```python
from build123d import *

# Parameters (mm, degrees)
SKETCH1_W           = 361.95
SKETCH1_H           = 460.375
BOSS_EXTRUDE1_DEPTH = 3.175
SKETCH2_W           = 3.175
SKETCH2_H           = 82.55
SKETCH2_H_2         = 44.45
SKETCH2_W_2         = 22.225
SKETCH2_H_3         = 3.175
CUT_EXTRUDE1_DEPTH  = 3.175
SKETCH3_R           = 12.0777
CUT_EXTRUDE2_DEPTH  = 3.175


with BuildPart() as part:
    # Sketch1 → Boss-Extrude1 (new body)
    with BuildSketch(Plane(origin=(0, 0, 0), x_dir=(0, 0, -1), z_dir=(1, 0, 0))):
        with Locations((0, 230.1875)):
            Rectangle(SKETCH1_W, SKETCH1_H)
    extrude(amount=BOSS_EXTRUDE1_DEPTH)

    # Sketch2 → Cut-Extrude1 (cut)
    with BuildSketch(Plane(origin=(3.175, 0, 0), x_dir=(0, 0, -1), z_dir=(1, 0, 0))):
        with Locations((-179.3875, 41.275)):
            Rectangle(SKETCH2_W, SKETCH2_H)
        with Locations((-179.3875, 180.975)):
            Rectangle(SKETCH2_W, SKETCH2_H_2)
        with Locations((-179.3875, 301.625)):
            Rectangle(SKETCH2_W, SKETCH2_H_2)
        Polygon((-98.425, 460.375), (-180.975, 460.375), (-180.975, 400.05), (-177.8, 400.05), (-177.8, 457.2), (-98.425, 457.2), align=None)
        with Locations((-11.1125, 458.7875)):
            Rectangle(SKETCH2_W_2, SKETCH2_H_3)
        with Locations((11.1125, 458.7875)):
            Rectangle(SKETCH2_W_2, SKETCH2_H_3)
        Polygon((180.975, 460.375), (98.425, 460.375), (98.425, 457.2), (177.8, 457.2), (177.8, 400.05), (180.975, 400.05), align=None)
        with Locations((179.3875, 301.625)):
            Rectangle(SKETCH2_W, SKETCH2_H_2)
        with Locations((179.3875, 180.975)):
            Rectangle(SKETCH2_W, SKETCH2_H_2)
        with Locations((179.3875, 41.275)):
            Rectangle(SKETCH2_W, SKETCH2_H)
    extrude(amount=-CUT_EXTRUDE1_DEPTH, mode=Mode.SUBTRACT)

    # Sketch3 → Cut-Extrude2 (cut)
    with BuildSketch(Plane(origin=(3.175, 0, 0), x_dir=(0, 0, -1), z_dir=(1, 0, 0))):
        with Locations((0, 50.8)):
            Circle(SKETCH3_R)
        with Locations((-90.5002, 50.8)):
            Circle(SKETCH3_R)
        with Locations((90.5002, 50.8)):
            Circle(SKETCH3_R)
    extrude(amount=-CUT_EXTRUDE2_DEPTH, mode=Mode.SUBTRACT)


solid = part.part
```
Work out the finished part from the listing and answer in its coordinate system (mm). Round coordinates to 2 decimals unless told otherwise and drop trailing zeros. Loops run counter-clockwise (first coordinate to the right, second up) from the corner with the lowest first, then second, coordinate; pieces in that order, holes last. Notation, with made-up numbers: M -31,-10 L 16,-10 A22 cw 16,18 Z; hole C 34,63.5 d8. An arc over 180 degrees is marked long. One line per question, with ' | ' between items.
Q1. Consider line 1 along Y through (x, z) = (0.75, 141); line 2 along Y through (x, z) = (3.05, 4); line 3 along Y through (x, z) = (2, 3). Determine where each line is inside the solid, lowest interval first. Write a range as from..to.
Conclusion:
line 1: y = 0..457.2 | line 2: y = 0..39.4, 62.2..457.2 | line 3: y = 0..39.1, 62.5..457.2
Q2. The mould has two halves that part along Y. Classify faces 1 (the flat face through (0, 233, 3)), 2 (the cylindrical face through (1.61, 51.331, 102.566)): +Y half, -Y half, draft (parallel to the pull), parting line (faces both ways), or undercut.
Conclusion:
face 1: draft | face 2: undercut
Q3. Find section B-B, the plane z = 0. Give the vertices of the cut face in (x, y) (3 decimals), then the cut area to 3 significant figures.
Conclusion:
outline: M 0,0 L 3.175,0 L 3.175,38.722 L 0,38.722 Z; M 0,62.878 L 3.175,62.878 L 3.175,457.2 L 0,457.2 Z | area: 1,370 mm2
Q4. Find section C-C, the plane x = 2.1. State how many separate pieces and enclosed holes the cut face has, then the cut area to 3 significant figures.
Conclusion:
separate pieces: 1 | enclosed holes: 3 | area: 163,000 mm2
Q5. Find section A-A, the plane y = 50.8. Give the vertices of the cut face in (x, z) (1 decimal), then the cut area to 3 significant figures.
Conclusion:
outline: M 0,-177.8 L 3.2,-177.8 L 3.2,-102.6 L 0,-102.6 Z; M 0,-78.4 L 3.2,-78.4 L 3.2,-12.1 L 0,-12.1 Z; M 0,12.1 L 3.2,12.1 L 3.2,78.4 L 0,78.4 Z; M 0,102.6 L 3.2,102.6 L 3.2,177.8 L 0,177.8 Z | area: 899 mm2
Q6. Each of these flat-tipped pins is pushed along its axis until it touches: pin 1 Ø1 at (x, z) = (1.5, -178.5) entering from +Y; pin 2 Ø1.6 at (x, y) = (1, 302.5) entering from -Z; pin 3 Ø1 at (x, z) = (2, 179) entering from -Y. Where does it stop, or does it pass through?
Conclusion:
pin 1: stops at y = 400.05 | pin 2: stops at z = -177.8 | pin 3: stops at y = 82.55
Q7. Find section D-D, the plane y = 177. Give the vertices of the cut face in (x, z) (3 decimals), then the cut area to 3 significant figures.
Conclusion:
outline: M 0,-177.8 L 3.175,-177.8 L 3.175,177.8 L 0,177.8 Z | area: 1,130 mm2
